```python
from build123d import *

# Parameters (mm, degrees)
F1_DEPTH = 43.084349


with BuildPart() as f1:
    # F0 (on Right) → F1 (new body)
    with BuildSketch(Plane.YZ):
        with BuildLine():
            ThreePointArc((0, -40.956058), (12.838283, -38.193702), (25.369942, -34.268193))
            Line((25.369942, -34.268193), (19.392215, -27.939987))
            Line((19.392215, -27.939987), (0, -40.956058))
        make_face()
        Polygon((19.392215, -27.939987), (25.369942, -34.268193), (40.151024, -23.927731), (25.369942, -23.927731), align=None)
        Polygon((-25.174692, 19.239914), (19.392215, -27.939987), (25.369942, -23.927731), (40.151024, -23.927731), (7.903695, 36.803901), align=None)
    extrude(amount=F1_DEPTH)


solid = f1.part
```
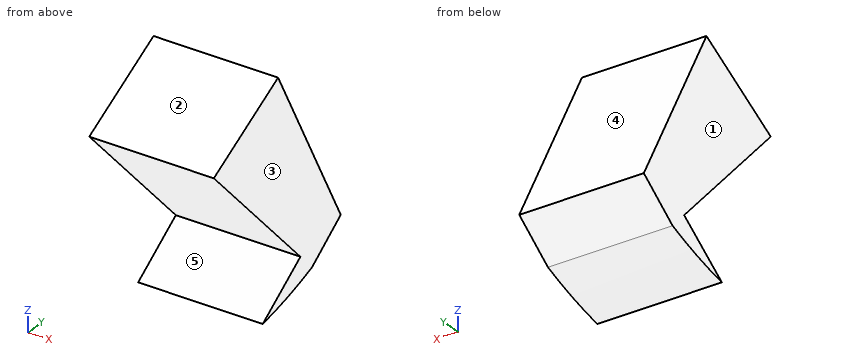
Verification items for the finished model (mm, model axes). Face numbers are marked on the shaded views. A direction names the side the tool comes from. Give positions to 0.01 mm unless a question says otherwise; leave off trailing zeros. Order: outer loops, then holes, each group sorted by start corner. A loop starts at its lowest first (then second) coordinate and runs counter-clockwise, first axis right, second up. Notation, with made-up numbers: (70, 61) -> (99, 61) arc R9 ccw to (99, 71) -> close; hole circle Ø3 at (51.5, 81.25). An arc over 180 degrees is marked (long way). One line per item, written item: value.
(1) Sectioned sample at D-D on y = 12. Record the cut outline in (x, z), then the cut area to 3 significant figures.
Final values:
outline: (0, -38.41) -> (43.08, -38.41) -> (43.08, -32.9) -> (0, -32.9) -> close; (0, -20.11) -> (43.08, -20.11) -> (43.08, 29.09) -> (0, 29.09) -> close
area: 2,360 mm^2
(2) Gauge pin test, flat ends, axial feed: pin 1 (6 mm diameter, centred on x = 19, y = -0.5, fed in from +Z); pin 2 (1.5 mm diameter, centred on x = 38.5, y = 13, fed in from +Z); pin 3 (2 mm diameter, centred on x = 27.5, z = 25, fed in from +Y). Record the tip position at first contact, or that the pin passes through.
Final values:
pin 1: z = 33.93
pin 2: z = 28.62
pin 3: y = 14.7
(3) Tool access check on the marked faces 4 and 5. Record the directions out of +Z, -Z, +X, -X, +Y, -Y that give a thin tool (end or side, any length) a straight path to the whole face; none if there is none.
Final values:
face 4: +Z, +X, -X, +Y
face 5: +X, -X, -Y
(4) Scan lines: line 1 along Z through (x, y) = (11, 3); line 2 along Z through (x, y) = (34, 9.5); line 3 along Z through (x, y) = (21, -13.5). Record each from-to range of solid material in increasing order. Write a range as [from, to].
Final values:
line 1: [-40.42, -38.94], [-10.59, 34.2]
line 2: [-39.03, -34.58], [-17.47, 33.8]
line 3: [6.88, 25.44]
(5) Sectioned sample at B-B on x = 35.5. Record the cut outline in (y, z), then the cut area to 3 significant figures.
Final values:
outline: (-25.17, 19.24) -> (19.39, -27.94) -> (0, -40.96) arc R143.36 ccw to (25.37, -34.27) -> (40.15, -23.93) -> (7.9, 36.8) -> close
area: 2,060 mm^2
(6) Sectioned sample at A-A on y = 1. Record the cut outline in (x, z), then the cut area to 3 significant figures.
Final values:
outline: (0, -40.78) -> (43.08, -40.78) -> (43.08, -40.28) -> (0, -40.28) -> close; (0, -8.47) -> (43.08, -8.47) -> (43.08, 33.14) -> (0, 33.14) -> close
area: 1,810 mm^2
(7) Draft check along X on the marked faces 1, 2 and 3. Enter one of: pulls with the +X half, pulls with the -X half, needs draft (parallel to the pull), parting line crosses it, or undercut.
Final values:
face 1: pulls with the -X half
face 2: needs draft
face 3: pulls with the +X half
(8) Sectioned sample at C-C on z = -9. Record the cut outline in (x, y), then the cut area to 3 significant figures.
Final values:
outline: (0, 1.5) -> (43.08, 1.5) -> (43.08, 32.22) -> (0, 32.22) -> close
area: 1,320 mm^2
